```python
from build123d import *

# Parameters (mm, degrees)
F0_R      = 30
F1_DEPTH  = 4
F2_R      = 6
F3_DEPTH  = 6
F4_R      = 1.5
F5_DEPTH  = 9.95
F6_W      = 4.6
F6_H      = 3
F7_DEPTH  = 9.4
F9_DEPTH  = 25
F11_DEPTH = 25


with BuildPart() as f1:
    # F0 (on Top) → F1 (new body)
    with BuildSketch(Plane.XY):
        Circle(F0_R)
    extrude(amount=F1_DEPTH)

    # F2 (on face) → F3 (join)
    with BuildSketch(Plane.XY.offset(4)):
        Circle(F2_R)
    extrude(amount=F3_DEPTH)

    # F4 (on Front) → F5 (cut, symmetric)
    with BuildSketch(Plane.XZ):
        with Locations((0, 7)):
            Circle(F4_R)
    extrude(amount=F5_DEPTH, both=True, mode=Mode.SUBTRACT)

    # F6 (on face) → F7 (cut)
    with BuildSketch(Plane.XY.offset(10)):
        Rectangle(F6_W, F6_H)
        with BuildLine():
            ThreePointArc((2.3, -1.5), (2.7459060435, 0), (2.3, 1.5))
            Line((2.3, 1.5), (2.3, -1.5))
        make_face()
        with BuildLine():
            Line((-2.3, -1.5), (-2.3, 1.5))
            ThreePointArc((-2.3, 1.5), (-2.7540939565, 0), (-2.3, -1.5))
        make_face()
    extrude(amount=-F7_DEPTH, mode=Mode.SUBTRACT)

    # F8 (on face) → F9 (cut)
    with BuildSketch(Plane.XY.offset(4)):
        with BuildLine():
            ThreePointArc((0, 16.5074747056), (-3.5121658528, 20.8878368139), (0, 25.2681989223))
            ThreePointArc((0, 25.2681989223), (-5.6994366386, 20.8878368139), (0, 16.5074747056))
        make_face()
        with BuildLine():
            ThreePointArc((-16.5074747056, 0), (-20.8878368139, -3.5121658528), (-25.2681989223, 0))
            ThreePointArc((-25.2681989223, 0), (-20.8878368139, -5.6994366386), (-16.5074747056, 0))
        make_face()
        with BuildLine():
            ThreePointArc((0, -16.5074747056), (3.5121658528, -20.8878368139), (0, -25.2681989223))
            ThreePointArc((0, -25.2681989223), (5.6994366386, -20.8878368139), (0, -16.5074747056))
        make_face()
        with BuildLine():
            ThreePointArc((16.5074747056, 0), (20.8878368139, 3.5121658528), (25.2681989223, 0))
            ThreePointArc((25.2681989223, 0), (20.8878368139, 5.6994366386), (16.5074747056, 0))
        make_face()
    extrude(amount=-F9_DEPTH, mode=Mode.SUBTRACT)

    # F10 (on face) → F11 (cut)
    with BuildSketch(Plane.XY.offset(4)):
        with BuildLine():
            ThreePointArc((-9.8298114426, 10.4183598849), (-9.7788159618, 10.8230928332), (-9.7617778379, 11.2306698208))
            ThreePointArc((-9.7617778379, 11.2306698208), (-9.9932757594, 12.7164090182), (-10.6658213511, 14.0612862161))
            Line((-10.6658213511, 14.0612862161), (-9.8298114426, 10.4183598849))
        make_face()
        with BuildLine():
            ThreePointArc((-10.6658213511, 14.0612862161), (-9.9932757594, 12.7164090182), (-9.7617778379, 11.2306698208))
            ThreePointArc((-9.7617778379, 11.2306698208), (-9.7788159618, 10.8230928332), (-9.8298114426, 10.4183598849))
            Line((-9.8298114426, 10.4183598849), (-7.759351705, 12.2398230505))
            Line((-7.759351705, 12.2398230505), (-10.6658213511, 14.0612862161))
        make_face()
        with BuildLine():
            Line((-13.8329075388, 16.0460758528), (-10.6658213511, 14.0612862161))
            ThreePointArc((-10.6658213511, 14.0612862161), (-12.0519648423, 15.3686673401), (-13.8329075388, 16.0460758528))
        make_face()
        Polygon((-9.8298114426, 10.4183598849), (-10.6658213511, 14.0612862161), (-13.8329075388, 16.0460758528), (-17.47583387, 15.2100659443), (-19.4606235067, 12.0429797567), (-18.6246135982, 8.4000534254), (-15.4575274105, 6.4152637887), (-11.8146010793, 7.2512736973), align=None)
        with BuildLine():
            ThreePointArc((-13.8329075388, 16.0460758528), (-12.0519648423, 15.3686673401), (-10.6658213511, 14.0612862161))
            Line((-10.6658213511, 14.0612862161), (-11.120263847, 16.8553626042))
            Line((-11.120263847, 16.8553626042), (-13.8329075388, 16.0460758528))
        make_face()
        with BuildLine():
            Line((-8.6883150478, 7.680528209), (-9.8298114426, 10.4183598849))
            ThreePointArc((-9.8298114426, 10.4183598849), (-10.5072199553, 8.6374171884), (-11.8146010793, 7.2512736973))
            Line((-11.8146010793, 7.2512736973), (-8.6883150478, 7.680528209))
        make_face()
        with BuildLine():
            ThreePointArc((-11.8146010793, 7.2512736973), (-10.5072199553, 8.6374171884), (-9.8298114426, 10.4183598849))
            Line((-9.8298114426, 10.4183598849), (-11.8146010793, 7.2512736973))
        make_face()
        with BuildLine():
            Line((-17.47583387, 15.2100659443), (-13.8329075388, 16.0460758528))
            ThreePointArc((-13.8329075388, 16.0460758528), (-15.7375170594, 15.9903824489), (-17.47583387, 15.2100659443))
        make_face()
        with BuildLine():
            ThreePointArc((-17.47583387, 15.2100659443), (-15.7375170594, 15.9903824489), (-13.8329075388, 16.0460758528))
            Line((-13.8329075388, 16.0460758528), (-16.2455738647, 17.609721433))
            Line((-16.2455738647, 17.609721433), (-17.47583387, 15.2100659443))
        make_face()
        with BuildLine():
            Line((-13.3300706432, 4.4496803728), (-11.8146010793, 7.2512736973))
            ThreePointArc((-11.8146010793, 7.2512736973), (-13.5529178899, 6.4709571926), (-15.4575274105, 6.4152637887))
            Line((-15.4575274105, 6.4152637887), (-13.3300706432, 4.4496803728))
        make_face()
        with BuildLine():
            ThreePointArc((-15.4575274105, 6.4152637887), (-13.5529178899, 6.4709571926), (-11.8146010793, 7.2512736973))
            Line((-11.8146010793, 7.2512736973), (-15.4575274105, 6.4152637887))
        make_face()
        with BuildLine():
            Line((-19.4606235067, 12.0429797567), (-17.47583387, 15.2100659443))
            ThreePointArc((-17.47583387, 15.2100659443), (-18.783214994, 13.8239224532), (-19.4606235067, 12.0429797567))
        make_face()
        with BuildLine():
            ThreePointArc((-19.4606235067, 12.0429797567), (-18.783214994, 13.8239224532), (-17.47583387, 15.2100659443))
            Line((-17.47583387, 15.2100659443), (-20.4682286884, 14.8799081511))
            Line((-20.4682286884, 14.8799081511), (-19.4606235067, 12.0429797567))
        make_face()
        with BuildLine():
            Line((-18.1701711023, 5.6059770373), (-15.4575274105, 6.4152637887))
            ThreePointArc((-15.4575274105, 6.4152637887), (-17.2384701071, 7.0926723014), (-18.6246135982, 8.4000534254))
            Line((-18.6246135982, 8.4000534254), (-18.1701711023, 5.6059770373))
        make_face()
        with BuildLine():
            ThreePointArc((-18.6246135982, 8.4000534254), (-17.2384701071, 7.0926723014), (-15.4575274105, 6.4152637887))
            Line((-15.4575274105, 6.4152637887), (-18.6246135982, 8.4000534254))
        make_face()
        with BuildLine():
            Line((-18.6246135982, 8.4000534254), (-19.4606235067, 12.0429797567))
            ThreePointArc((-19.4606235067, 12.0429797567), (-19.4049301028, 10.138370236), (-18.6246135982, 8.4000534254))
        make_face()
        with BuildLine():
            ThreePointArc((-18.6246135982, 8.4000534254), (-19.4049301028, 10.138370236), (-19.4606235067, 12.0429797567))
            Line((-19.4606235067, 12.0429797567), (-21.1133740596, 9.7463018969))
            Line((-21.1133740596, 9.7463018969), (-18.6246135982, 8.4000534254))
        make_face()
        Polygon((-14.8799081511, -20.4682286884), (-12.0429797567, -19.4606235067), (-9.7463018969, -21.1133740596), (-8.4000534254, -18.6246135982), (-5.6059770373, -18.1701711023), (-6.4152637887, -15.4575274105), (-4.4496803728, -13.3300706432), (-7.2512736973, -11.8146010793), (-7.680528209, -8.6883150478), (-10.4183598849, -9.8298114426), (-12.2398230505, -7.759351705), (-14.0612862161, -10.6658213511), (-16.8553626042, -11.120263847), (-16.0460758528, -13.8329075388), (-17.609721433, -16.2455738647), (-15.2100659443, -17.47583387), align=None)
        Polygon((20.4682286884, -14.8799081511), (19.4606235067, -12.0429797567), (21.1133740596, -9.7463018969), (18.6246135982, -8.4000534254), (18.1701711023, -5.6059770373), (15.4575274105, -6.4152637887), (13.3300706432, -4.4496803728), (11.8146010793, -7.2512736973), (8.6883150478, -7.680528209), (9.8298114426, -10.4183598849), (7.759351705, -12.2398230505), (10.6658213511, -14.0612862161), (11.120263847, -16.8553626042), (13.8329075388, -16.0460758528), (16.2455738647, -17.609721433), (17.47583387, -15.2100659443), align=None)
        Polygon((14.8799081511, 20.4682286884), (12.0429797567, 19.4606235067), (9.7463018969, 21.1133740596), (8.4000534254, 18.6246135982), (5.6059770373, 18.1701711023), (6.4152637887, 15.4575274105), (4.4496803728, 13.3300706432), (7.2512736973, 11.8146010793), (7.680528209, 8.6883150478), (10.4183598849, 9.8298114426), (12.2398230505, 7.759351705), (14.0612862161, 10.6658213511), (16.8553626042, 11.120263847), (16.0460758528, 13.8329075388), (17.609721433, 16.2455738647), (15.2100659443, 17.47583387), align=None)
    extrude(amount=-F11_DEPTH, mode=Mode.SUBTRACT)

    # F12 (on Front) → F13 (revolve, cut)
    with BuildSketch(Plane.XZ):
        Polygon((30, 0.5857864376), (30, 3.4142135624), (28.5857864376, 2), align=None)
    revolve(axis=Axis((0, 0, 3.4037481528), (0, 0, 1)), mode=Mode.SUBTRACT)


solid = f1.part
```
CAD build for the part. Positions are in the model's coordinates, mm. A direction names the side the tool comes from. Round coordinates to 2 decimals unless told otherwise and drop trailing zeros. Order: outer loops, then holes, each group sorted by start corner. A loop starts at its lowest first (then second) coordinate and runs counter-clockwise, first axis right, second up.
Q1. Drop flat-ended pins along their axis: pin 1 (3 mm diameter, centred on x = -3, z = 4.5, fed in from -Y); pin 2 (8 mm diameter, centred on x = 1.17, y = -20.89, fed in from -Z); pin 3 (4 mm diameter, centred on y = 2.5, z = 7, fed in from -X); pin 4 (12 mm diameter, centred on x = -20.89, y = -1.17, fed in from +Z). Give the stop position or say it passes through.
Q2. Slice it at A-A (z = 7). Write the cut outline in (x, y), and give its area (3 significant figures).
Q3. Which spindle directions (+Z, -Z, +X, -X, +Y, -Y) get a long thin tool onto all of the face, cutting with end or side? Do faces 1 (the flat face through (0, -1.5, 5)), 2 (the flat face through (19.97, -13.48, 2.03)). Say none if no direction does.
Q4. Wall check: L1, parallel to Y at x = -16, z = 1; L2, parallel to X at y = 11.5, z = 2.75; L3, parallel to Z at x = 0, y = -3.7. Give the ranges that are in metal, low to high.
Results below:
1. pin 1: stops at y = -29.96
1. pin 2: stops at z = 0
1. pin 3: stops at x = -5.98
1. pin 4: stops at z = 4
2. outline: (-2.3, -1.5) arc R2.7 cw to (-2.3, 1.5) - (-1.5, 1.5) - (-1.5, 5.81) arc R6 ccw to (-1.5, -5.81) - (-1.5, -1.5) - close; (1.5, -5.81) arc R6 ccw to (1.5, 5.81) - (1.5, 1.5) - (2.3, 1.5) arc R2.75 cw to (2.3, -1.5) - (1.5, -1.5) - close
2. area: 70.8 mm2
3. face 1: +Z
3. face 2: +Z, -Z
4. L1: y = -24.89 to -17.07, -10.98 to 6.25, 17.45 to 24.89
4. L2: x = -26.99 to -19.85, -8.6 to 7.29, 16.74 to 26.99
4. L3: z = 0 to 5.5, 8.5 to 10
